Geometry: final body of the model. Coordinates: model frame, mm. A direction names the side the tool comes from. Round coordinates to 2 decimals unless told otherwise and drop trailing zeros. Loops run counter-clockwise (first coordinate to the right, second up) from the corner with the lowest first, then second, coordinate; pieces in that order, holes last. Notation, with made-up numbers: (-1.5, -11) - (17.5, -11) arc R23 cw to (17.5, 24) - close; hole circle Ø4 at (45, -35). An arc over 180 degrees is marked (long way). Return JSON: item names as keys, results as strings. Group by question number.
1. Section C-C on x = 19. Return loops of the section in (y, z), and give its area (3 significant figures).
2. Section A-A on y = 2.15. Return loops of the section in (x, z).
3. First-contact query: pin 1 Ø0.9 at (y, z) = (4, -6.5) entering from +X; pin 2 Ø5.5 at (x, z) = (16, -37) entering from +Y; pin 3 Ø1 at (y, z) = (3, -36) entering from -X. Flat tips, straight axial feed; report the tip coordinate or a pass-through.
4. Set-up query: faces 4 (the face through (16, 3, -25)), 5 (the face through (19.8, 3, -36)), 6 (the face through (25.5, 3, -12)), 7 (the face through (16, 3.7, -37)), 8 (the face through (6.5, 3, -12)). Return all of +Z, -Z, +X, -X, +Y, -Y with unobstructed straight access to the full face (end or side cutting, diameter ignored); none if empty.
5. Draft query along Z for faces 1 (the face through (16, 2, 0)), 2 (the face through (12.2, 3, -36)), 3 (the face through (16, 3, -34)). Return one class per face: +Z half, -Z half, draft (parallel to the pull), parting line (faces both ways), or undercut.
6. Material intervals for probe 1 along Z at (x, y) = (12.5, 2.55); probe 2 along Y at (x, z) = (17.5, -25.5); probe 3 along Y at (x, z) = (14.5, -36), sorted ascending.
7. Section B-B on z = -13. Return loops of the section in (x, y).
8. Section D-D on z = -28.5. Return loops of the section in (x, y), and give its area (3 significant figures).
from build123d import *

# Parameters (mm, degrees)
SKETCH1_W           = 32
SKETCH1_H           = 39
BOSS_EXTRUDE1_DEPTH = 1.7
CHAMFER1_SIZE       = 2
SKETCH3_W           = 19
SKETCH3_H           = 25
BOSS_EXTRUDE2_DEPTH = 3
SKETCH4_W           = 7.6
SKETCH4_H           = 5
BOSS_EXTRUDE3_DEPTH = 2


with BuildPart() as part:
    # Sketch1 → Boss-Extrude1 (new body)
    with BuildSketch(Plane(origin=(0, 0, 0), x_dir=(1, 0, 0), z_dir=(0, 1, 0))):
        with Locations((16, 19.5)):
            Rectangle(SKETCH1_W, SKETCH1_H)
    extrude(amount=BOSS_EXTRUDE1_DEPTH)

    # Chamfer1
    chamfer1_edges = [part.edges().sort_by_distance(p)[0] for p in [
        (32, 0.85, 0),
        (0, 0.85, 0),
    ]]
    chamfer(chamfer1_edges, length=CHAMFER1_SIZE)

    # Sketch3 → Boss-Extrude2 (add)
    with BuildSketch(Plane(origin=(0, 1.7, 0), x_dir=(1, 0, 0), z_dir=(0, 1, 0))):
        with Locations((16, 12.5)):
            Rectangle(SKETCH3_W, SKETCH3_H)
    extrude(amount=BOSS_EXTRUDE2_DEPTH)

    # Sketch4 → Boss-Extrude3 (add)
    with BuildSketch(Plane(origin=(0, 1.7, 0), x_dir=(1, 0, 0), z_dir=(0, 1, 0))):
        with Locations((16, 36.5)):
            Rectangle(SKETCH4_W, SKETCH4_H)
    extrude(amount=BOSS_EXTRUDE3_DEPTH)


solid = part.part
Taken from the geometry:
{
 "1": {"outline": "(0, -39) - (3.7, -39) - (3.7, -34) - (1.7, -34) - (1.7, -25) - (4.7, -25) - (4.7, 0) - (0, 0) - close", "area": "151 mm2"},
 "2": {"outline": "(6.5, -25) - (25.5, -25) - (25.5, 0) - (6.5, 0) - close; (12.2, -39) - (19.8, -39) - (19.8, -34) - (12.2, -34) - close"},
 "3": {"pin 1": "x = 25.5", "pin 2": "y = 3.7", "pin 3": "x = 12.2"},
 "4": {"face 4": "+X, -X, +Y", "face 5": "-Z, +X, +Y", "face 6": "+Z, -Z, +X, +Y", "face 7": "-Z, +X, -X, +Y", "face 8": "+Z, -Z, -X, +Y"},
 "5": {"face 1": "+Z half", "face 2": "draft", "face 3": "undercut"},
 "6": {"probe 1": "-39 to -34, -25 to 0", "probe 2": "0 to 1.7", "probe 3": "0 to 3.7"},
 "7": {"outline": "(0, 0) - (32, 0) - (32, 1.7) - (25.5, 1.7) - (25.5, 4.7) - (6.5, 4.7) - (6.5, 1.7) - (0, 1.7) - close"},
 "8": {"outline": "(0, 0) - (32, 0) - (32, 1.7) - (0, 1.7) - close", "area": "54.4 mm2"}
}
